Build history of the part. All positions in model axes, mm. Give positions to 0.01 mm unless a question says otherwise; leave off trailing zeros. Loops run counter-clockwise (first coordinate to the right, second up) from the corner with the lowest first, then second, coordinate; pieces in that order, holes last.
1) Flat gauge pins, fed straight in: P1, Ø1, axis at x = 12, y = -34.5, coming from the -Z side; P2, Ø1.5, axis at y = -51, z = -12, coming from the -X side. Where does each tip first touch, or does it go through?
2) Band-saw the part on C-C on z = -10.65. List the corners of the cut face in (x, y), then the cut area to 3 significant figures.
3) Band-saw the part on A-A on y = -31. List the corners of the cut face in (x, z).
4) Wall check: line 1 (X direction, y = -52, z = -11.75). Give the ranges that are in metal, low to high.
5) Band-saw the part on B-B on x = 4. List the corners of the cut face in (y, z), then the cut area to 3 significant figures.
```python
from build123d import *

# Parameters (mm, degrees)
F1_DEPTH   = 70
F2_SIZE2   = 3
F2_SIZE    = 1
F3_SIZE2   = 1
F3_SIZE    = 3
F3_2_SIZE2 = 1
F3_2_SIZE  = 3


with BuildPart() as f1:
    # F0 (on Front) → F1 (new body)
    with BuildSketch(Plane.XZ):
        Polygon((13.2, -10.2), (0, -10.2), (0, -13), (11.2, -13), (11.2, -11.6), (13.2, -11.6), align=None)
        Polygon((0, -13), (0, -10.2), (-13.2, -10.2), (-13.2, -11.6), (-11.2, -11.6), (-11.2, -13), align=None)
    extrude(amount=F1_DEPTH)

    # F2
    f2_edges = [f1.edges().sort_by_distance(p)[0] for p in [
        (0, -70, -13),
        (0, -70, -10.2),
    ]]
    f2_side = f1.faces().sort_by_distance((0, -70, -11.542623))[0]
    chamfer(f2_edges, length=F2_SIZE, length2=F2_SIZE2, reference=f2_side)

    # F3
    f3_edges = [f1.edges().sort_by_distance(p)[0] for p in [
        (0, 0, -10.2),
    ]]
    f3_side = f1.faces().sort_by_distance((0, -33.5, -10.2))[0]
    chamfer(f3_edges, length=F3_SIZE, length2=F3_SIZE2, reference=f3_side)

    # F3#2
    f3_2_edges = [f1.edges().sort_by_distance(p)[0] for p in [
        (0, 0, -13),
    ]]
    f3_2_side = f1.faces().sort_by_distance((0, -33.5, -13))[0]
    chamfer(f3_2_edges, length=F3_2_SIZE, length2=F3_2_SIZE2, reference=f3_2_side)


solid = f1.part
```
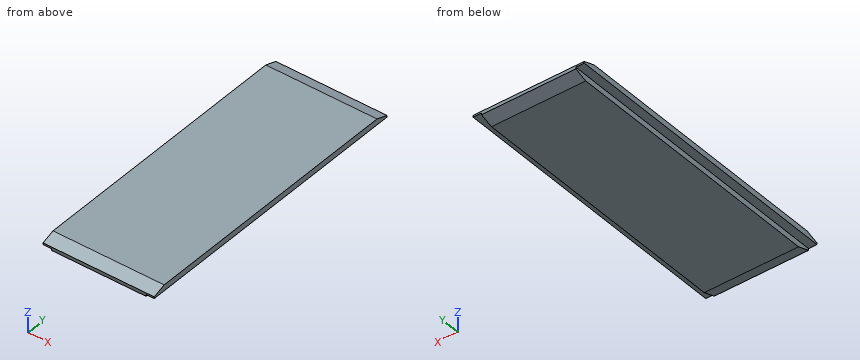
Findings below:
1. P1: stops at z = -11.6
1. P2: stops at x = -13.2
2. outline: (-13.2, -68.35) - (13.2, -68.35) - (13.2, -1.65) - (-13.2, -1.65) - close
2. area: 1,760 mm2
3. outline: (-13.2, -11.6) - (-11.2, -11.6) - (-11.2, -13) - (11.2, -13) - (11.2, -11.6) - (13.2, -11.6) - (13.2, -10.2) - (-13.2, -10.2) - close
4. line 1: x = -11.2 to 11.2
5. outline: (-70, -12) - (-67, -13) - (-3, -13) - (0, -12) - (0, -11.2) - (-3, -10.2) - (-67, -10.2) - (-70, -11.2) - close
5. area: 190 mm2
